from build123d import *

# Parameters (mm, degrees)
SKETCH1_R           = 3.4
SKETCH1_R_2         = 5
SKETCH1_R_3         = 8
SKETCH1_R_4         = 1.5
SKETCH1_R_5         = 6
BOSS_EXTRUDE1_DEPTH = 3
SKETCH4_R           = 1.5
CUT_EXTRUDE1_DEPTH  = 3
CIRPATTERN1_COUNT   = 6


with BuildPart() as part:
    # Sketch1 → Boss-Extrude1 (new body)
    with BuildSketch(Plane.XY):
        with BuildLine():
            ThreePointArc((-271.800817077, 243.790124811), (-269.253440252, 250.876511464), (-272.371911597, 257.730790488))
            Line((-272.371911597, 257.730790488), (-308.701287129, 292.107311249))
            ThreePointArc((-308.701287129, 292.107311249), (-315.968083296, 294.835963731), (-322.997699137, 291.544099213))
            ThreePointArc((-322.997699137, 291.544099213), (-376.789694918, 217.612042952), (-413.944817586, 134.07148626))
            ThreePointArc((-413.944817586, 134.07148626), (-413.283077207, 126.337537039), (-407.288017737, 121.406904946))
            Line((-407.288017737, 121.406904946), (-359.356506069, 107.119186605))
            ThreePointArc((-359.356506069, 107.119186605), (-351.861081548, 107.843490223), (-346.996122098, 113.591374532))
            ThreePointArc((-346.996122098, 113.591374532), (-316.172961568, 182.603306357), (-271.800817077, 243.790124811))
        make_face()
        with Locations((-373.746213466, 131.27857223)):
            Circle(SKETCH1_R, mode=Mode.SUBTRACT)
        with Locations((-371.824242114, 147.162716089)):
            Circle(SKETCH1_R_2, mode=Mode.SUBTRACT)
        with Locations((-369.902270762, 163.046859947)):
            Circle(SKETCH1_R, mode=Mode.SUBTRACT)
        with Locations((-310.189407893, 252.536198061)):
            Circle(SKETCH1_R_3, mode=Mode.SUBTRACT)
        with Locations((-326.120312176, 219.178644843)):
            Circle(SKETCH1_R_4, mode=Mode.SUBTRACT)
        with Locations((-339.543705934, 195.928644843)):
            Circle(SKETCH1_R_4, mode=Mode.SUBTRACT)
        with Locations((-352.967099693, 219.178644843)):
            Circle(SKETCH1_R_4, mode=Mode.SUBTRACT)
        with Locations((-339.543705934, 218.428644843)):
            Circle(SKETCH1_R_5, mode=Mode.SUBTRACT)
    extrude(amount=BOSS_EXTRUDE1_DEPTH)

    # Sketch4 → Cut-Extrude1 (cut)
    with BuildSketch(Plane.XY.offset(3)):
        with Locations((-324.043705934, 211.428644843)):
            Circle(SKETCH4_R)
    cut_extrude1 = extrude(amount=-CUT_EXTRUDE1_DEPTH, mode=Mode.SUBTRACT)

    # CirPattern1: Cut-Extrude1 ×6 about axis
    cirpattern1_axis = Axis((-339.543705934, 211.428644843, 0), (0, 0, 1))
    for i in range(1, CIRPATTERN1_COUNT):
        add(cut_extrude1.rotate(cirpattern1_axis, i * 360 / CIRPATTERN1_COUNT), mode=Mode.SUBTRACT)


solid = part.part
Check sheet for the modelled part. Datum: model origin and axes. Units: mm. Round coordinates to 2 decimals unless told otherwise and drop trailing zeros. Order: outer loops, then holes, each group sorted by start corner. A loop starts at its lowest first (then second) coordinate and runs counter-clockwise, first axis right, second up. Notation, with made-up numbers: M 63,-27.75 L 104,-27.75 A8 cw 104,-22.75 Z; hole C 48.5,-24.5 d10. An arc over 180 degrees is marked long. One line per item, written item: value. Start each with the question number.
1. Gauge pin test, flat ends, axial feed: P1, Ø3.5, axis at x = -324.04, y = 211.43, coming from the +Z side; P2, Ø1, axis at x = -337, z = 1.5, coming from the -Y side. Record the tip position at first contact, or that the pin passes through.
2. Scan lines: line 1 along X through (y, z) = (199, 2.6); line 2 along Y through (x, z) = (-317, 0.8); line 3 along Y through (x, z) = (-352, 2). Record each from-to range of solid material in increasing order.
3. Section check D-D on y = 179.5. Enter the section's corners in (x, z).
4. Section check A-A on z = 1.95. Give the number of separate pieces and of enclosed holes in the cut face, and give its area (3 significant figures).
5. Section check C-C on x = -391. Enter the section's corners in (y, z).
6. Release check for a two-part mould opening along Y. For faces 1 (the flat face through (-343, 202, 3)), 2 (the cylindrical face through (-372.18, 128.26, 1.48)), 3 (the flat face through (-383.658, 114.363, 1.479)) record: released by +Y, released by -Y, zero draft, split by the parting line, or undercut.
7. Section check B-B on y = 215. Enter the section's corners in (x, z), and give its area (3 significant figures).
Results found:
1. P1: z = 3
1. P2: y = 139.29
2. line 1: -386.94 to -348.42, -346.17 to -332.92, -330.67 to -306.12
2. line 2: 181.16 to 248.34, 256.73 to 294.74
2. line 3: 107.77 to 218.03, 220.33 to 255.78
3. outline: M -396.37,0 L -317.95,0 L -317.95,3 L -396.37,3 Z
4. separate pieces: 1
4. enclosed holes: 14
4. area: 12,500 mm^2
5. outline: M 116.55,0 L 190.9,0 L 190.9,3 L 116.55,3 Z
6. face 1: zero draft
6. face 2: undercut
6. face 3: released by -Y
7. outline: M -378.29,0 L -344.47,0 L -344.47,3 L -378.29,3 Z; M -334.62,0 L -295.1,0 L -295.1,3 L -334.62,3 Z
7. area: 220 mm^2
